Part print with two shaded views. Sizes in mm from the minimum x, y, z corner. A direction names the side the tool comes from. Coordinates: 2 decimals unless noted, no trailing zeros. Write each loop counter-clockwise with the first axis right and the second up, starting at its lowest first coordinate (ties: lowest second). Pieces come first, ordered by that corner, then holes. Notation, with made-up numbers: (-13.5, 41.5) - (9.5, 41.5) arc R16 ccw to (9.5, 68.5) - close; hole circle Ø6 at (-36, 19). An arc over 180 degrees is marked (long way). One line per question, with ' | ' between items. Start each with the question number.
1. Band-saw the part on D-D, the plane z = 16.5. Write the cut outline in (x, y), then the cut area to 3 significant figures.
2. Two-plate mould, pull along Z, no slides. Class the marked faces 1, 2 and 3: +Z half, -Z half, draft (parallel to the pull), parting line (faces both ways), or undercut.
3. Which spindle directions (+Z, -Z, +X, -X, +Y, -Y) get a long thin tool onto all of the face, cutting with end or side? Do the marked faces 4, 5, 6 and 7. Say none if no direction does.
4. Band-saw the part on B-B, the plane y = 24.5. Write the cut outline in (x, z).
5. Flat gauge pins, fed straight in: P1, Ø5, axis at y = 71, z = 3.5, coming from the -X side; P2, Ø3, axis at x = 46.5, y = 54.5, coming from the -Z side; P3, Ø4, axis at x = 60, z = 7.5, coming from the -Y side. Where does each tip first touch, or does it go through?
6. Probe line 1 (Z direction, x = 41, y = 64.5); line 2 (Y direction, x = 18, z = 19.25); line 3 (Z direction, x = 23, y = 74). List the from-to ranges inside material, lowest first.
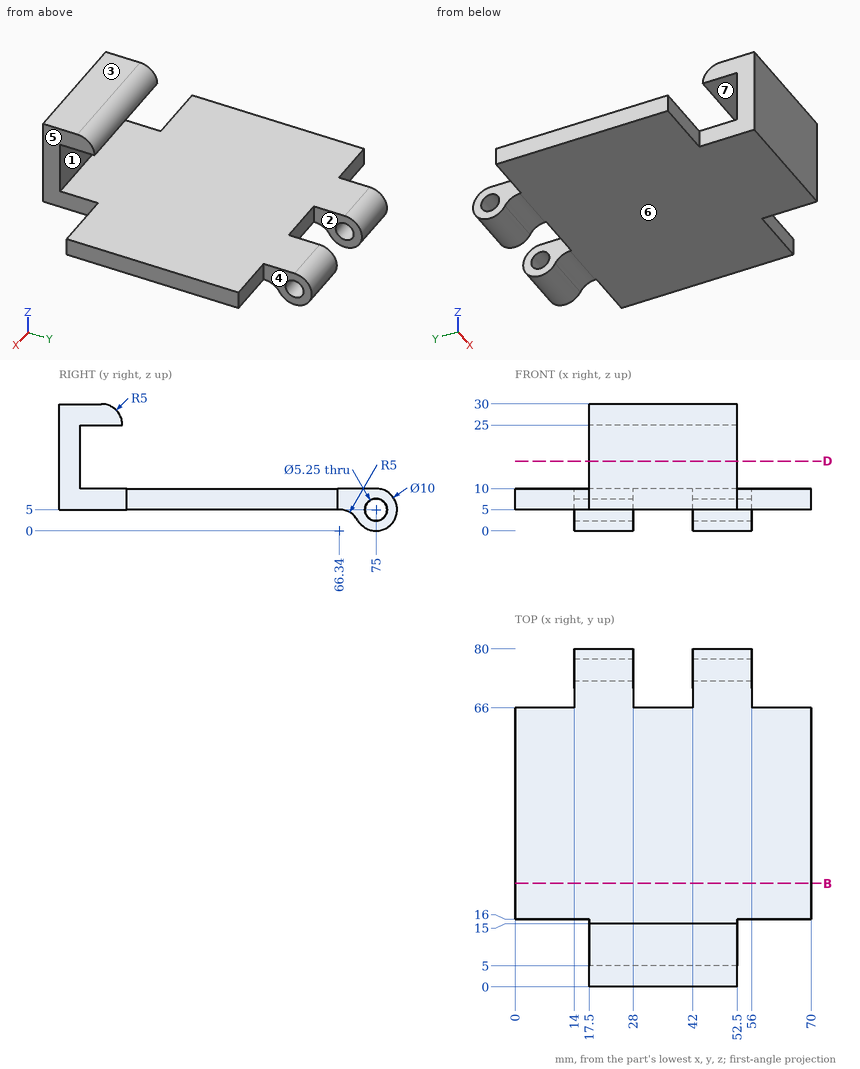
Filled in:
1) outline: (17.5, 0) - (52.5, 0) - (52.5, 5) - (17.5, 5) - close | area: 175 mm²
2) face 1: undercut | face 2: draft | face 3: +Z half
3) face 4: +Z, -Z, +X, +Y | face 5: +Z, -Z, +X, -Y | face 6: -Z, +X, -X, -Y | face 7: +X, -X, +Y
4) outline: (0, 5) - (70, 5) - (70, 10) - (0, 10) - close
5) P1: stops at x = 14 | P2: stops at z = 5 | P3: stops at y = 16
6) line 1: z = 5 to 10 | line 2: y = 0 to 5 | line 3: z = 0.1 to 2.57, 7.43 to 10
